Build history of the part. All positions in model axes, mm. A direction names the side the tool comes from. Round coordinates to 2 decimals unless told otherwise and drop trailing zeros. Order: outer loops, then holes, each group sorted by start corner. A loop starts at its lowest first (then second) coordinate and runs counter-clockwise, first axis right, second up. Notation, with made-up numbers: (14.25, 83) - (53.25, 83) arc R17 ccw to (53.25, 112) - close; hole circle Ø5 at (11, 47). An arc over 180 degrees is marked (long way). Write each question's results on one line, items separated by ' | '. Start each with the question number.
```python
from build123d import *

# Parameters (mm, degrees)
SKETCH029_W          = 6.25
SKETCH029_H          = 6.25
PAD018_DEPTH         = 15
THICKNESS005_T       = 1
SKETCH030_W          = 1.75
SKETCH030_H          = 2
SKETCH030_W_2        = 3
SKETCH030_H_2        = 3
POCKET006_DEPTH      = 1.126
POCKET006_DEPTH_BACK = 7.126


with BuildPart() as part:
    # Sketch029 → Pad018 (new body)
    with BuildSketch(Plane.XY):
        Rectangle(SKETCH029_W, SKETCH029_H)
    extrude(amount=PAD018_DEPTH)

    # Thickness005
    thickness005_openings = [part.faces().sort_by_distance(p)[0] for p in [
        (0, 0, 15),
        (0, 0, 0),
    ]]
    offset(amount=THICKNESS005_T, openings=thickness005_openings)

    # Sketch030 → Pocket006 (cut, two sides)
    with BuildSketch(Plane.XZ.offset(3)) as pocket006_sk:
        with Locations((-2.25, 1)):
            Rectangle(SKETCH030_W, SKETCH030_H)
        with Locations((2.25, 1)):
            Rectangle(SKETCH030_W, SKETCH030_H)
        with Locations((0, 6.5)):
            Rectangle(SKETCH030_W_2, SKETCH030_H_2)
    extrude(amount=POCKET006_DEPTH, mode=Mode.SUBTRACT)
    extrude(pocket006_sk.sketch, amount=-POCKET006_DEPTH_BACK, mode=Mode.SUBTRACT)


solid = part.part
```
1. Mould opens along Y. For faces 1 (the face through (-1.375, 3.6, 1)), 2 (the face through (3.125, 0, 7)), 3 (the face through (3.84, 3.824, 7.605)) say: pulls with the +Y half, pulls with the -Y half, needs draft (parallel to the pull), parting line crosses it, or undercut.
2. 3-axis set-ups, long thin cutter, end or side, ignore diameter. For faces 4 (the face through (0, 3.125, 9)), 5 (the face through (-1.5, -3.6, 6.5)), 6 (the face through (1.375, -3.6, 1)), 7 (the face through (-3.84, 3.824, 7.605)), 8 (the face through (0, 3.6, 0)): which of +Z, -Z, +X, -X, +Y, -Y reach the whole face in a straight line?
3. Flat gauge pins, fed straight in: pin 1 Ø0.5 at (x, y) = (-2, 4) entering from -Z; pin 2 Ø4 at (x, y) = (1.5, -1) entering from +Z; pin 3 Ø0.8 at (y, z) = (4, 1) entering from -X (3 decimals). Where does each tip first touch, or does it go through?
4. Cut at D-D (x = 0.5). List the corners of the cut face in (y, z) (3 decimals).
5. Cut at B-B (x = 2). List the corners of the cut face in (y, z) (3 decimals), plus the area to 3 significant figures.
6. Cut at A-A (y = 2). List the corners of the cut face in (x, z) (3 decimals).
7. Cut at C-C (z = 9). List the corners of the cut face in (x, y) (3 decimals).
8. Wall check: line 1 (X direction, y = -3, z = 4) (3 decimals); line 2 (Z direction, x = -0.5, y = -3.25). Give the ranges that are in metal, low to high. Write a range as from..to.
A:
1) face 1: needs draft | face 2: undercut | face 3: pulls with the +Y half
2) face 4: +Z, -Z | face 5: +Y, -Y | face 6: -Z, +Y, -Y | face 7: +Z, -Z, -X, +Y | face 8: -Z, +X, -X, +Y, -Y
3) pin 1: stops at z = 2 | pin 2: stops at z = 15 | pin 3: stops at x = -4.005
4) outline: (-4.125, 0) - (-3.125, 0) - (-3.125, 5) - (-4.125, 5) - close; (-4.125, 8) - (-3.125, 8) - (-3.125, 15) - (-4.125, 15) - close; (3.125, 0) - (4.125, 0) - (4.125, 5) - (3.125, 5) - close; (3.125, 8) - (4.125, 8) - (4.125, 15) - (3.125, 15) - close
5) outline: (-4.125, 2) - (-3.125, 2) - (-3.125, 15) - (-4.125, 15) - close; (3.125, 2) - (4.125, 2) - (4.125, 15) - (3.125, 15) - close | area: 26.0 mm^2
6) outline: (-4.125, 0) - (-3.125, 0) - (-3.125, 15) - (-4.125, 15) - close; (3.125, 0) - (4.125, 0) - (4.125, 15) - (3.125, 15) - close
7) outline: (-4.125, -3.125) arc R1 ccw to (-3.125, -4.125) - (3.125, -4.125) arc R1 ccw to (4.125, -3.125) - (4.125, 3.125) arc R1 ccw to (3.125, 4.125) - (-3.125, 4.125) arc R1 ccw to (-4.125, 3.125) - close; hole (-3.125, -3.125) - (3.125, -3.125) - (3.125, 3.125) - (-3.125, 3.125) - close
8) line 1: x = -4.125..-3.125, 3.125..4.125 | line 2: z = 0..5, 8..15
